```python
from build123d import *

# Parameters (mm, degrees)
F1_DEPTH = 2.8


with BuildPart() as f1:
    # F0 (on Front) → F1 (new body)
    with BuildSketch(Plane.XZ):
        with BuildLine():
            ThreePointArc((4.45, 11.4), (0, 6.95), (-4.45, 11.4))
            Line((-4.45, 11.4), (-4.45, 2.8))
            Line((-4.45, 2.8), (-2.35, 2.8))
            Line((-2.35, 2.8), (-2.35, 0))
            Line((-2.35, 0), (-2.95, 0))
            Line((-2.95, 0), (-2.95, -0.5))
            Line((-2.95, -0.5), (-3.65, -0.5))
            Line((-3.65, -0.5), (-2.55, -4.5))
            Line((-2.55, -4.5), (2.55, -4.5))
            Line((2.55, -4.5), (3.65, -0.5))
            Line((3.65, -0.5), (2.95, -0.5))
            Line((2.95, -0.5), (2.95, 0))
            Line((2.95, 0), (2.35, 0))
            Line((2.35, 0), (2.35, 2.8))
            Line((2.35, 2.8), (4.45, 2.8))
            Line((4.45, 2.8), (4.45, 11.4))
        make_face()
        with BuildLine():
            ThreePointArc((-0.55, 1.45), (0, 2), (0.55, 1.45))
            Line((0.55, 1.45), (0.55, -1.45))
            ThreePointArc((0.55, -1.45), (0, -2), (-0.55, -1.45))
            Line((-0.55, -1.45), (-0.55, 1.45))
        make_face(mode=Mode.SUBTRACT)
    extrude(amount=F1_DEPTH)


solid = f1.part
```
Here's how the part is built. I have some questions about the finished solid (model axes, mm). A direction names the side the tool comes from. Coordinates: 2 decimals unless noted, no trailing zeros. Order: outer loops, then holes, each group sorted by start corner. A loop starts at its lowest first (then second) coordinate and runs counter-clockwise, first axis right, second up. Notation, with made-up numbers: (19, -22) - (33, -22) arc R23 cw to (33, 17) - close; hole circle Ø5 at (10.25, 50.5). An arc over 180 degrees is marked (long way). One line per question, with ' | ' between items.
(1) If we mould it in two halves opening along X, with no side actions, what happens to faces 4 (the flat face through (-4.45, -1, 7)), 5 (the flat face through (2.35, -1, 1)), 6 (the cylindrical face through (0, -1, 2))? For each: pulls with the +X half, pulls with the -X half, needs draft (parallel to the pull), parting line crosses it, or undercut.
Report:
face 4: pulls with the -X half | face 5: pulls with the +X half | face 6: undercut
(2) If I drill on L1, parallel to X at y = -0.2, z = 0.25; L2, parallel to Z at x = -2.5, y = -0.1, over which ranges is the centre line in solid material (lowest first)?
Report:
L1: x = -2.35 to -0.55, 0.55 to 2.35 | L2: z = -4.5 to 0, 2.8 to 7.72
(3) Suppose I cut it at C-C on z = -1. List the corners of the cut face in (x, y) for me, and give its area (3 significant figures).
Report:
outline: (-3.51, -2.8) - (-0.55, -2.8) - (-0.55, 0) - (-3.51, 0) - close; (0.55, -2.8) - (3.51, -2.8) - (3.51, 0) - (0.55, 0) - close | area: 16.6 mm2
(4) Suppose I cut it at A-A on x = 0. List the corners of the cut face in (y, z) for me.
Report:
outline: (-2.8, -4.5) - (0, -4.5) - (0, -2) - (-2.8, -2) - close; (-2.8, 2) - (0, 2) - (0, 6.95) - (-2.8, 6.95) - close
(5) Suppose I cut it at B-B on y = -1.6. List the corners of the cut face in (x, z) for me, and give its area (3 significant figures).
Report:
outline: (-4.45, 2.8) - (-2.35, 2.8) - (-2.35, 0) - (-2.95, 0) - (-2.95, -0.5) - (-3.65, -0.5) - (-2.55, -4.5) - (2.55, -4.5) - (3.65, -0.5) - (2.95, -0.5) - (2.95, 0) - (2.35, 0) - (2.35, 2.8) - (4.45, 2.8) - (4.45, 11.4) arc R4.45 cw to (-4.45, 11.4) - close; hole (-0.55, -1.45) arc R0.55 ccw to (0.55, -1.45) - (0.55, 1.45) arc R0.55 ccw to (-0.55, 1.45) - close | area: 82.2 mm2
(6) For faces 1 (the flat face through (-2.35, -1, 1)), 2 (the flat face through (3, -1, 2.8)), 3 (the flat face through (0.55, -1, 0)), which set-ups out of +Z, -Z, +X, -X, +Y, -Y let a thin tool reach every point of the face, with its end or its side?
Report:
face 1: -X, +Y, -Y | face 2: +X, +Y, -Y | face 3: +Y, -Y
(7) Will these pins go through, and if not, where does the flat tip stop? pin 1 (0.6 mm diameter, centred on y = -2, z = 0, fed in from -X); pin 2 (0.5 mm diameter, centred on x = -2.5, y = -1, fed in from +Z).
Report:
pin 1: stops at x = -2.95 | pin 2: stops at z = 7.9
